For this review, take the finished solid that the model builds, in its own axes (mm). Face numbers are marked on the shaded views. A direction names the side the tool comes from. Round coordinates to 2 decimals unless told otherwise and drop trailing zeros. Write each loop counter-clockwise with the first axis right and the second up, starting at its lowest first coordinate (ties: lowest second). Pieces come first, ordered by that corner, then holes. Notation, with made-up numbers: (49.5, 77) -> (64.5, 77) arc R22 cw to (64.5, 116) -> close; hole circle Ø2 at (73, 9). An arc over 180 degrees is marked (long way). Answer in a Markdown table with one row per item.
from build123d import *

# Parameters (mm, degrees)
SKETCH_1_W                          = 105
SKETCH_1_H                          = 158
EXTRUDE_1_DEPTH                     = 10
CUT_EXTRUDE_1_REACH                 = 97.38
SKETCH_2_R                          = 6.5
CHAMFER_1_SIZE                      = 5.5
CHAMFER_1_SIZE2                     = 7
PATTERN_LINEAR_1_COUNT              = 2
PATTERN_LINEAR_1_PITCH              = 70
CHAMFER_1_OF_PATTERN_LINEAR_1_SIZE2 = 7
CHAMFER_1_OF_PATTERN_LINEAR_1_SIZE  = 5.5
CUT_EXTRUDE_2_REACH                 = 133.78
SKETCH_4_W                          = 45
SKETCH_4_H                          = 158
CUT_EXTRUDE_3_DEPTH                 = 6


with BuildPart() as part:
    # 草图1 → 凸台-拉伸1 (new body)
    with BuildSketch(Plane(origin=(0, 0, 0), x_dir=(1, 0, 0), z_dir=(0, 1, 0))):
        Rectangle(SKETCH_1_W, SKETCH_1_H)
    extrude(amount=EXTRUDE_1_DEPTH)

    # 草图2 → 切除-拉伸1 (cut, up to next)
    with BuildSketch(Plane.XZ, mode=Mode.PRIVATE) as cut_extrude_1_sk1:
        with Locations(Location((17.5, 35, 0), (0, 0, 270))):
            Circle(SKETCH_2_R)
    cut_extrude_1_tool1 = extrude(cut_extrude_1_sk1.sketch, amount=-CUT_EXTRUDE_1_REACH, mode=Mode.PRIVATE) & part.part
    cut_extrude_1 = cut_extrude_1_tool1.solids().sort_by_distance((17.5, 0, 35))[0]
    add(cut_extrude_1, mode=Mode.SUBTRACT)

    # 倒角1
    chamfer_1_edges = [part.edges().sort_by_distance(p)[0] for p in [
        (17.5, 0, 41.5),
    ]]
    chamfer_1_side = [part.faces().sort_by_distance(p)[0] for p in [
        (-0.141142206, 0, -0.282284412),
    ]]
    chamfer(chamfer_1_edges, length=CHAMFER_1_SIZE, length2=CHAMFER_1_SIZE2, reference=chamfer_1_side[0])

    # 阵列(线性)1: 切除-拉伸1 ×2
    with Locations(*[(0, 0, -i * PATTERN_LINEAR_1_PITCH) for i in range(1, PATTERN_LINEAR_1_COUNT)]):
        add(cut_extrude_1, mode=Mode.SUBTRACT)

    # 倒角1 of 阵列(线性)1
    chamfer_1_of_pattern_linear_1_edges = [part.edges().sort_by_distance(p)[0] for p in [
        (17.5, 0, -28.5),
    ]]
    chamfer(chamfer_1_of_pattern_linear_1_edges, length=CHAMFER_1_OF_PATTERN_LINEAR_1_SIZE, length2=CHAMFER_1_OF_PATTERN_LINEAR_1_SIZE2)

    # 草图3 → 切除-拉伸2 (cut, up to next)
    with BuildSketch(Plane(origin=(52.5, 0, 0), x_dir=(0, 0, -1), z_dir=(1, 0, 0)), mode=Mode.PRIVATE) as cut_extrude_2_sk1:
        Polygon((-79, 10), (-79, 0), (-75.000285359, 10), align=None)
    cut_extrude_2_tool1 = extrude(cut_extrude_2_sk1.sketch, amount=-CUT_EXTRUDE_2_REACH, mode=Mode.PRIVATE) & part.part
    # 草图3 → 切除-拉伸2 (cut, up to next)
    with BuildSketch(Plane(origin=(52.5, 0, 0), x_dir=(0, 0, -1), z_dir=(1, 0, 0)), mode=Mode.PRIVATE) as cut_extrude_2_sk2:
        Polygon((79, 10), (79, 0), (75.000285359, 10), align=None)
    cut_extrude_2_tool2 = extrude(cut_extrude_2_sk2.sketch, amount=-CUT_EXTRUDE_2_REACH, mode=Mode.PRIVATE) & part.part
    add(cut_extrude_2_tool1.solids().sort_by_distance((52.5, 6.666667, 77.666762))[0], mode=Mode.SUBTRACT)
    add(cut_extrude_2_tool2.solids().sort_by_distance((52.5, 6.666667, -77.666762))[0], mode=Mode.SUBTRACT)

    # 草图4 → 切除-拉伸3 (cut)
    with BuildSketch(Plane(origin=(0, 10, 0), x_dir=(1, 0, 0), z_dir=(0, 1, 0))):
        with Locations((-30, 0)):
            Rectangle(SKETCH_4_W, SKETCH_4_H)
    extrude(amount=-CUT_EXTRUDE_3_DEPTH, mode=Mode.SUBTRACT)


solid = part.part
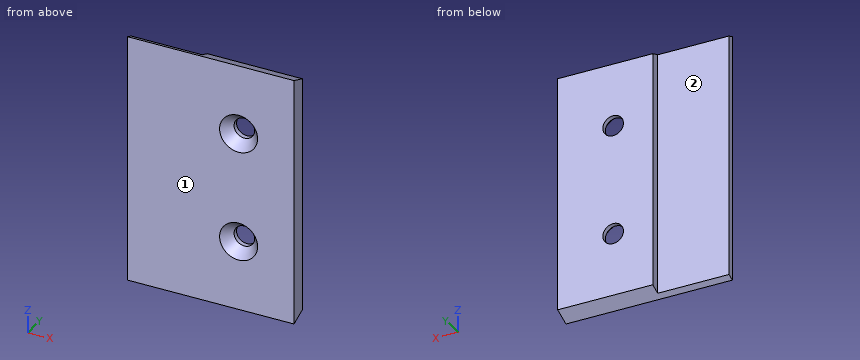
1) Consider section C-C on y = 2.25. State the section outline as (x, z) points.
Solved:
| item | result |
|---|---|
| outline | (-52.5, -78.1) -> (52.5, -78.1) -> (52.5, 78.1) -> (-52.5, 78.1) -> close; hole circle Ø20.46 at (17.5, -35); hole circle Ø20.46 at (17.5, 35) |
2) For the marked faces 1 and 2, list the 3-axis set-ups (+Z, -Z, +X, -X, +Y, -Y) from which the entire face can be reached by the end or side of a thin tool; tool diameter is ignored.
Solved:
| item | result |
|---|---|
| face 1 | +Z, -Z, +X, -X, -Y |
| face 2 | +Z, -Z, -X, +Y |
3) Clearance check with flat-ended pins moving along their axes: pin 1 Ø8 at (x, z) = (17.5, 35) entering from -Y (3 decimals); pin 2 Ø5 at (x, y) = (38, 3.5) entering from -Z; pin 3 Ø3 at (x, z) = (-23.5, -1) entering from +Y; pin 4 Ø2 at (x, y) = (-40, 2) entering from +Z. State where each tip first meets the part, or that it passes through.
Solved:
| item | result |
|---|---|
| pin 1 | through |
| pin 2 | z = -78.6 |
| pin 3 | y = 4 |
| pin 4 | z = 78.6 |
4) Consider section B-B on z = -35. State the section outline as (x, y) points, then the cut area to 4 significant figures.
Solved:
| item | result |
|---|---|
| outline | (-52.5, 0) -> (5.5, 0) -> (11, 7) -> (11, 10) -> (-7.5, 10) -> (-7.5, 4) -> (-52.5, 4) -> close; (24, 7) -> (29.5, 0) -> (52.5, 0) -> (52.5, 10) -> (24, 10) -> close |
| area | 611.5 mm² |
5) Consider section A-A on x = 17.5. State the section outline as (y, z) points, then the cut area to 3 significant figures.
Solved:
| item | result |
|---|---|
| outline | (0, -79) -> (10, -75) -> (10, -41.5) -> (7, -41.5) -> (0, -47) -> close; (0, -23) -> (7, -28.5) -> (10, -28.5) -> (10, 28.5) -> (7, 28.5) -> (0, 23) -> close; (0, 47) -> (7, 41.5) -> (10, 41.5) -> (10, 75) -> (0, 79) -> close |
| area | 1,200 mm² |
6) For line 1 (X direction, y = 7.8, z = -35); line 2 (Z direction, x = 11.5, y = 2.5); line 3 (X direction, y = 8, z = -15), list the stretches that pass through material, from the lowest coordinate up. Write a range as [from, to].
Solved:
| item | result |
|---|---|
| line 1 | [-7.5, 11], [24, 52.5] |
| line 2 | [-78, -43.04], [-26.96, 26.96], [43.04, 78] |
| line 3 | [-7.5, 52.5] |
7) Consider section D-D on z = -54.5. State the section outline as (x, y) points, then the cut area to 3 significant figures.
Solved:
| item | result |
|---|---|
| outline | (-52.5, 0) -> (52.5, 0) -> (52.5, 10) -> (-7.5, 10) -> (-7.5, 4) -> (-52.5, 4) -> close |
| area | 780 mm² |
